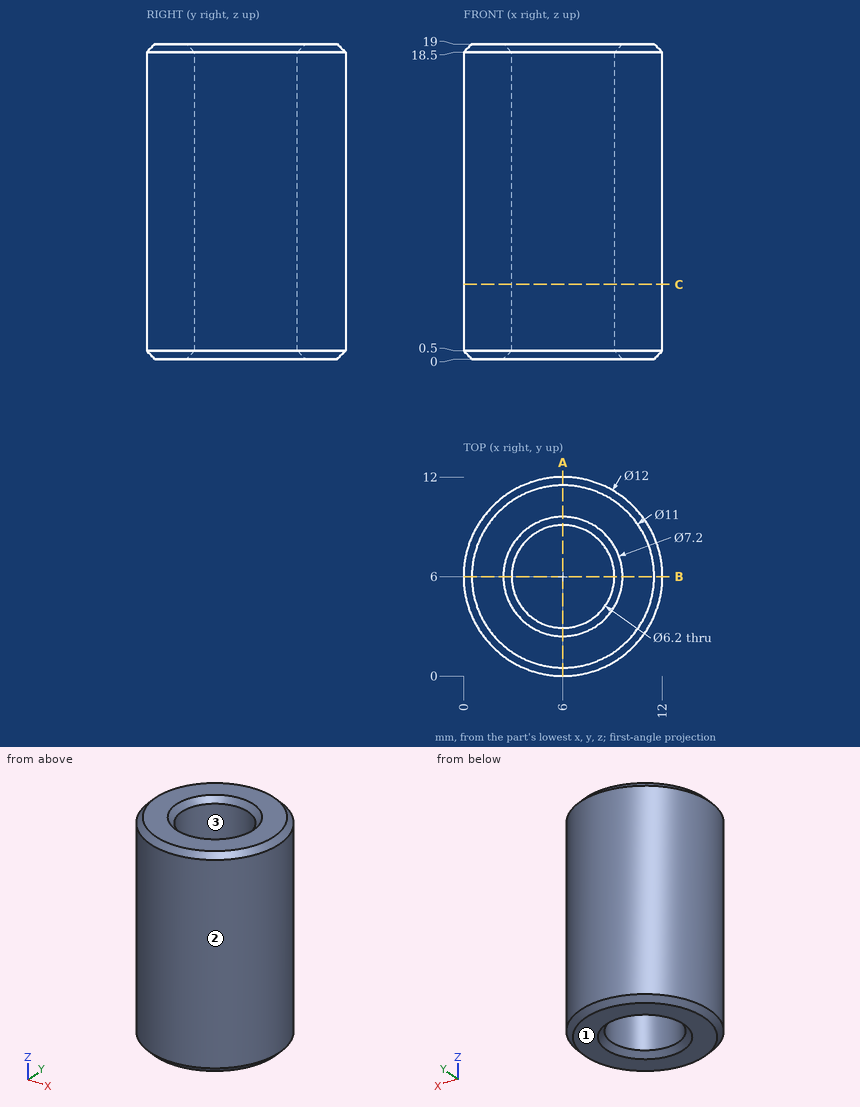
Print and shaded views of the part. All mm, measured from the part's lowest x, y and z. Give positions to 0.01 mm unless a question says otherwise; leave off trailing zeros. Loops run counter-clockwise (first coordinate to the right, second up) from the corner with the lowest first, then second, coordinate; pieces in that order, holes last.
1) Pull direction Y, two halves, no side cores. Call the marked faces 1, 2 and 3: +Y half, -Y half, draft (parallel to the pull), parting line (faces both ways), or undercut.
2) Flat gauge pin, fed straight in: pin 1 Ø2 at (x, y) = (9, 6) entering from -Z. Where does the tip first touch, or does it go through?
3) Wall check: line 1 (Y direction, x = 6, z = 8.75); line 2 (Y direction, x = 4.5, z = 16); line 3 (X direction, y = 3.5, z = 1.25). Give the ranges that are in metal, low to high.
4) Saw through at A-A (x = 6). Write the cut outline in (y, z).
5) Saw through at C-C (z = 4.5). Write the cut outline in (x, y), plus the area to 3 significant figures.
Answer block:
1. face 1: draft
1. face 2: parting line
1. face 3: undercut
2. pin 1: stops at z = 0
3. line 1: y = 0 to 2.9, 9.1 to 12
3. line 2: y = 0.19 to 3.29, 8.71 to 11.81
3. line 3: x = 0.55 to 4.17, 7.83 to 11.45
4. outline: (0, 0.5) - (0.5, 0) - (2.4, 0) - (2.9, 0.5) - (2.9, 18.5) - (2.4, 19) - (0.5, 19) - (0, 18.5) - close; (9.1, 0.5) - (9.6, 0) - (11.5, 0) - (12, 0.5) - (12, 18.5) - (11.5, 19) - (9.6, 19) - (9.1, 18.5) - close
5. outline: circle Ø12 at (6, 6); hole circle Ø6.2 at (6, 6)
5. area: 82.9 mm2
